Build history of the part. All positions in model axes, mm. A direction names the side the tool comes from. Round coordinates to 2 decimals unless told otherwise and drop trailing zeros. Order: outer loops, then holes, each group sorted by start corner. A loop starts at its lowest first (then second) coordinate and runs counter-clockwise, first axis right, second up. Notation, with made-up numbers: M 74.25,15.25 L 93.25,15.25 A26 ccw 93.25,53.25 Z; hole C 89.25,0 d7. An arc over 180 degrees is marked long. Use CSV: the item, a comma, the result in double quotes.
from build123d import *

# Parameters (mm, degrees)
PAD_DEPTH       = 10
SKETCH001_W     = 25
SKETCH001_H     = 50
POCKET_DEPTH    = 5
SKETCH002_R     = 2
POCKET001_DEPTH = 12
FILLET_R        = 2
FILLET001_R     = 1
POCKET002_DEPTH = 5
SKETCH004_W     = 40
SKETCH004_H     = 30
POCKET003_DEPTH = 5


with BuildPart() as part:
    # Sketch → Pad (new body)
    with BuildSketch(Plane.XY):
        with BuildLine():
            Line((-25, 0), (0, 0))
            Line((0, 0), (0, 40))
            Line((0, 40), (-75, 40))
            Line((-75, 40), (-75, 35))
            Line((-75, 35), (-67, 35))
            Line((-67, 35), (-67, 15))
            Line((-67, 15), (-75, 15))
            Line((-75, 15), (-75, 10))
            add(Edge.make_bspline(
                [(-25, 0), (-25, 10), (-75, 10)],
                knots=[0, 0, 0, 1, 1, 1], degree=2))
        make_face()
    extrude(amount=PAD_DEPTH)

    # Sketch001 → Pocket (cut)
    with BuildSketch(Plane.XY):
        with Locations((-7.5, 20)):
            Rectangle(SKETCH001_W, SKETCH001_H)
    extrude(amount=POCKET_DEPTH, mode=Mode.SUBTRACT)

    # Sketch002 → Pocket001 (cut)
    with BuildSketch(Plane.XY):
        with Locations((-8, 30)):
            Circle(SKETCH002_R)
        with Locations((-8, 10)):
            Circle(SKETCH002_R)
    extrude(amount=POCKET001_DEPTH, mode=Mode.SUBTRACT)

    # Fillet
    fillet_edges = [part.edges().sort_by_distance(p)[0] for p in [
        (0, 40, 7.5),
        (0, 0, 7.5),
        (-75, 10, 5),
        (-75, 40, 5),
    ]]
    fillet(fillet_edges, radius=FILLET_R)

    # Fillet001
    fillet001_edges = [part.edges().sort_by_distance(p)[0] for p in [
        (-25, 0, 5),
    ]]
    fillet(fillet001_edges, radius=FILLET001_R)

    # Sketch003 (on Face13 of Fillet001) → Pocket002 (cut)
    with BuildSketch(Plane(origin=(0, 40, 0), x_dir=(-1, 0, 0), z_dir=(0, 1, 0))):
        Polygon((65, -5), (65, 5), (60, 5), (60, 15), (55, 15), (55, 5), (50, 5), (50, -5), align=None)
        Polygon((45, -5), (45, 5), (40, 5), (40, 15), (35, 15), (35, 5), (30, 5), (30, -5), align=None)
    extrude(amount=-POCKET002_DEPTH, mode=Mode.SUBTRACT)

    # Sketch004 (on Face5 of Pocket002) → Pocket003 (cut)
    with BuildSketch(Plane(origin=(0, 0, 0), x_dir=(1, 0, 0), z_dir=(0, 0, -1))):
        with Locations((-40, -15)):
            Rectangle(SKETCH004_W, SKETCH004_H)
    extrude(amount=-POCKET003_DEPTH, mode=Mode.SUBTRACT)


solid = part.part
(1) Cut at B-B, the plane z = 8.75. Count the separate pieces of the cut face and the enclosed holes in it, and give its area (3 significant figures).
Answer block:
separate pieces,"1"
enclosed holes,"2"
area,"2,340 mm²"
(2) Wall check: line 1 (Y direction, x = -8, z = 8.9); line 2 (Z direction, x = -3, y = 16.5); line 3 (Y direction, x = -39, z = 1). Give the ranges that are in metal, low to high. Write a range as from..to.
Answer block:
line 1,"y = 0..8, 12..28, 32..40"
line 2,"z = 5..10"
line 3,"y = 30..35"
(3) Two-plate mould, pull along X, no slides. Class faces 5 (the face through (-30, 20, 10)), 6 (the face through (-30, 38, 3)), 7 (the face through (-0.6, 0.57, 7.54)): released by +X, released by -X, zero draft, split by the parting line, or undercut.
Answer block:
face 5,"zero draft"
face 6,"undercut"
face 7,"released by +X"
(4) Cut at A-A, the plane x = -8. Give the cut face in (y, z).
Answer block:
outline,"M 0,5 L 8,5 L 8,10 L 0,10 Z; M 12,5 L 28,5 L 28,10 L 12,10 Z; M 32,5 L 40,5 L 40,10 L 32,10 Z"
(5) Tool access for faces 1 (the face through (-71, 15, 5)), 2 (the face through (-40, 30, 2)), 3 (the face through (-20, 35, 2)), 4 (the face through (-55, 38, 8)): list every direction of +Z, -Z, +X, -X, +Y, -Y with a clear straight run to the whole face (end or side of a thin tool).
Answer block:
face 1,"+Z, -Z, -X"
face 2,"-Z, +X, -Y"
face 3,"-Z, +X, +Y, -Y"
face 4,"+Z, -Z, +Y"
(6) Drop flat-ended pins along their axis: pin 1 (5.5 mm diameter, centred on y = 37, z = 2, fed in from +X); pin 2 (4 mm diameter, centred on x = -31.5, z = 2.5, fed in from -Y); pin 3 (3 mm diameter, centred on y = 27, z = 7.5, fed in from -X); pin 4 (6.5 mm diameter, centred on x = -8, y = 30, fed in from +Z). Give the stop position or say it passes through.
Answer block:
pin 1,"stops at x = -20"
pin 2,"stops at y = 30"
pin 3,"stops at x = -67"
pin 4,"stops at z = 10"
